Check sheet for the modelled part. Datum: model origin and axes. Units: mm. A direction names the side the tool comes from. Coordinates: 2 decimals unless noted, no trailing zeros. Loops run counter-clockwise (first coordinate to the right, second up) from the corner with the lowest first, then second, coordinate; pieces in that order, holes last. Notation, with made-up numbers: M 49.5,-26.5 L 62.5,-26.5 A20 ccw 62.5,-9.5 Z; hole C 1,-0.5 d7. An arc over 180 degrees is marked long. Return JSON: item names as keys, results as strings.
from build123d import *

# Parameters (mm, degrees)
PAD_DEPTH    = 26
POCKET_DEPTH = 6


with BuildPart() as part:
    # Sketch → Pad (new body)
    with BuildSketch(Plane.XY):
        with BuildLine():
            ThreePointArc((-13.266499, 20), (0, 12), (13.266499, 20))
            Line((13.266499, 20), (16.266499, 20))
            Line((16.266499, 20), (16.266499, 0))
            Line((-16.266499, 0), (16.266499, 0))
            Line((-16.266499, 20), (-16.266499, 0))
            Line((-13.266499, 20), (-16.266499, 20))
        make_face()
    extrude(amount=PAD_DEPTH)

    # Sketch001 → Pocket (cut)
    with BuildSketch(Plane.XZ):
        Polygon((4, 6.071797), (8, 13), (4, 19.928203), (-4, 19.928203), (-8, 13), (-4, 6.071797), align=None)
    extrude(amount=-POCKET_DEPTH, mode=Mode.SUBTRACT)


solid = part.part
1) Section check D-D on x = 0. Record the cut outline in (y, z).
Answers:
{"outline": "M 0,0 L 12,0 L 12,26 L 0,26 L 0,19.93 L 6,19.93 L 6,6.07 L 0,6.07 Z"}
2) Section check C-C on y = 17.75. Record the cut outline in (x, z), then the cut area to 3 significant figures.
Answers:
{"outline": "M -16.27,0 L -11.81,0 L -11.81,26 L -16.27,26 Z; M 11.81,0 L 16.27,0 L 16.27,26 L 11.81,26 Z", "area": "232 mm²"}
3) Go/stop test with flat-tipped pins: pin 1 Ø3 at (x, z) = (-2.5, 11.5) entering from -Y; pin 2 Ø5 at (x, z) = (-6.5, 9.5) entering from +Y. Record where each tip stops, or that it passes through.
Answers:
{"pin 1": "y = 6", "pin 2": "y = 15"}
4) Section check A-A on y = 4.5. Record the cut outline in (x, z).
Answers:
{"outline": "M -16.27,0 L 16.27,0 L 16.27,26 L -16.27,26 Z; hole M -8,13 L -4,6.07 L 4,6.07 L 8,13 L 4,19.93 L -4,19.93 Z"}
5) Scan lines: line 1 along X through (y, z) = (17.5, 14.5); line 2 along X through (y, z) = (14.5, 10.75); line 3 along Y through (x, z) = (0, 15.75). Record each from-to range of solid material in increasing order. Write a range as [from, to].
Answers:
{"line 1": "[-16.27, -11.61], [11.61, 16.27]", "line 2": "[-16.27, -8.29], [8.29, 16.27]", "line 3": "[6, 12]"}
6) Set-up check for faces 4 (the face through (-6.028, 2.958, 9.584)), 5 (the face through (-15, 20, 13)): record each of +Z, -Z, +X, -X, +Y, -Y from which the full face is reachable in a straight line by a thin tool's end or side.
Answers:
{"face 4": "-Y", "face 5": "+Z, -Z, +X, -X, +Y"}
7) Section check B-B on z = 22.25. Record the cut outline in (x, y).
Answers:
{"outline": "M -16.27,0 L 16.27,0 L 16.27,20 L 13.27,20 A15 cw -13.27,20 L -16.27,20 Z"}
8) Draft check along X on faces 1 (the face through (16.266, 10, 13)), 2 (the face through (0, 3, 6.072)), 3 (the face through (-7, 0, 16)). Enter one of: +X half, -X half, draft (parallel to the pull), parting line (faces both ways), or undercut.
Answers:
{"face 1": "+X half", "face 2": "undercut", "face 3": "draft"}
